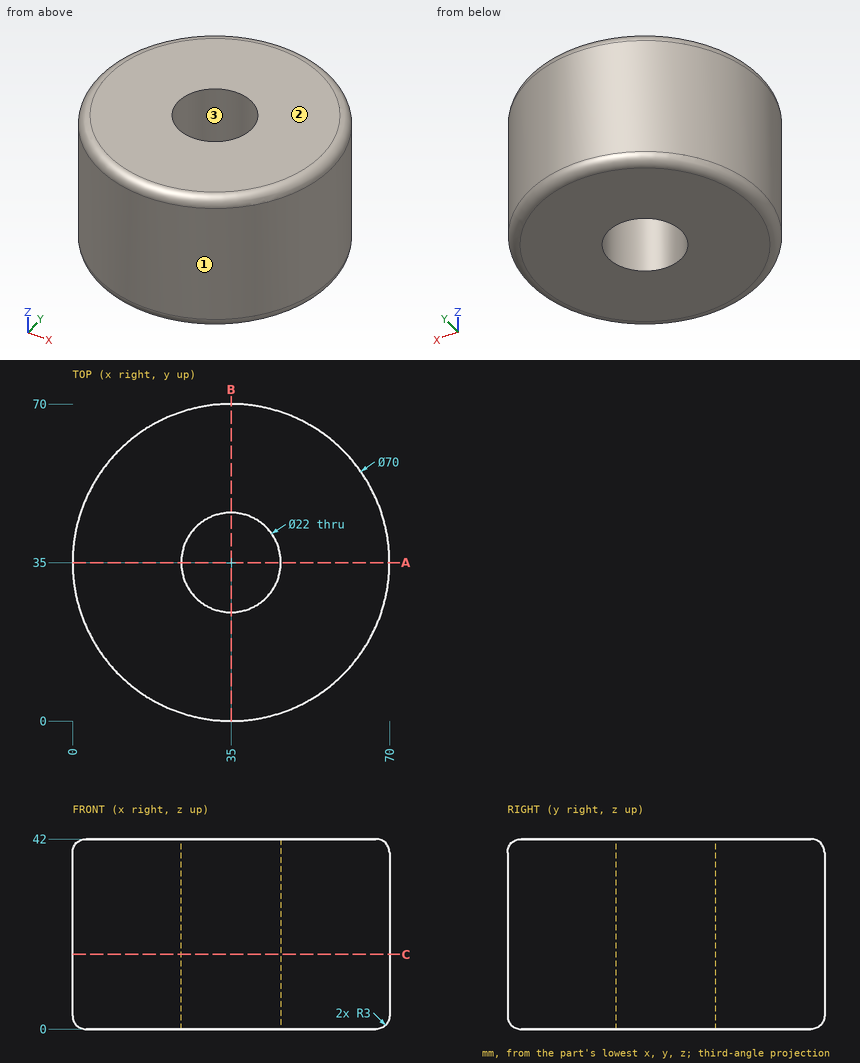
Geometry check sheet. Reference: drawing and pictorial views, mm from the part's lowest x, y, z. Coordinates: 2 decimals unless noted, no trailing zeros. Write each loop counter-clockwise with the first axis right and the second up, starting at its lowest first coordinate (ties: lowest second). Pieces come first, ordered by that corner, then holes. Notation, with made-up numbers: M 13.25,47 L 29.25,47 A14 cw 29.25,55 Z; hole C 41.25,71 d3. An arc over 180 degrees is marked long. Write item = value, one per line. Start each with the question number.
1. Thickness scan on probe 1 along Y at (x, z) = (35, 19.5); probe 2 along X at (y, z) = (32.5, 27); probe 3 along X at (y, z) = (26.5, 36). Record the ranges inside material, lowest first.
2. Sectioned sample at C-C (z = 16.5). Record the cut outline in (x, y).
3. Mould release check, pull along Y, two halves, no side actions. Record for the marked faces 1, 2 and 3: pulls with the +Y half, pulls with the -Y half, needs draft (parallel to the pull), parting line crosses it, or undercut.
4. Sectioned sample at A-A (y = 35). Record the cut outline in (x, z), then the cut area to 3 significant figures.
5. Go/stop test with flat-tipped pins: pin 1 (1 mm diameter, centred on y = 35.5, z = 18.5, fed in from +X); pin 2 (12 mm diameter, centred on y = 10, z = 35.5, fed in from -X); pin 3 (8 mm diameter, centred on x = 37.5, z = 10, fed in from -Y); pin 4 (3 mm diameter, centred on y = 9, z = 4.5, fed in from -X) (3 decimals). Record where each tip stops, or that it passes through.
The answers:
q1.probe_1 = 0 to 24, 46 to 70
q1.probe_2 = 0.09 to 24.29, 45.71 to 69.91
q1.probe_3 = 1.05 to 28.02, 41.98 to 68.95
q2.outline = C 35,35 d70; hole C 35,35 d22
q3.face_1 = parting line crosses it
q3.face_2 = needs draft
q3.face_3 = undercut
q4.outline = M 0,3 A3 ccw 3,0 L 24,0 L 24,42 L 3,42 A3 ccw 0,39 Z; M 46,0 L 67,0 A3 ccw 70,3 L 70,39 A3 ccw 67,42 L 46,42 Z
q4.area = 2,010 mm²
q5.pin_1 = 70
q5.pin_2 = 5.61
q5.pin_3 = 0
q5.pin_4 = 10.005
